```python
from build123d import *

# Parameters (mm, degrees)
F0_R     = 10
F0_W     = 40
F0_H     = 20
F1_DEPTH = 30


with BuildPart() as f1:
    # F0 (on Front) → F1 (new body)
    with BuildSketch(Plane.XZ):
        with BuildLine():
            Line((0, 20), (0, 0))
            Line((0, 0), (110, 0))
            ThreePointArc((110, 0), (117.071068, 2.928932), (120, 10))
            ThreePointArc((120, 10), (122.928932, 17.071068), (130, 20))
            Line((130, 20), (140, 20))
            ThreePointArc((140, 20), (147.071068, 22.928932), (150, 30))
            Line((150, 30), (150, 110))
            ThreePointArc((150, 110), (147.071068, 117.071068), (140, 120))
            Line((140, 120), (130, 120))
            ThreePointArc((130, 120), (122.928932, 122.928932), (120, 130))
            ThreePointArc((120, 130), (117.071068, 137.071068), (110, 140))
            Line((110, 140), (10, 140))
            ThreePointArc((10, 140), (2.928932, 137.071068), (0, 130))
            ThreePointArc((0, 130), (-2.928932, 122.928932), (-10, 120))
            Line((-10, 120), (-40, 120))
            ThreePointArc((-40, 120), (-47.071068, 117.071068), (-50, 110))
            Line((-50, 110), (-50, 30))
            ThreePointArc((-50, 30), (-47.071068, 22.928932), (-40, 20))
            Line((-40, 20), (0, 20))
        make_face()
        with BuildLine():
            Line((-40, 30), (-40, 50))
            Line((-40, 50), (0, 50))
            Line((0, 50), (0, 40))
            ThreePointArc((0, 40), (-2.928932, 32.928932), (-10, 30))
            Line((-10, 30), (-40, 30))
        make_face(mode=Mode.SUBTRACT)
        with BuildLine():
            Line((20, 30), (20, 70))
            Line((20, 70), (100, 70))
            Line((100, 70), (100, 30))
            ThreePointArc((100, 30), (97.071068, 22.928932), (90, 20))
            Line((90, 20), (30, 20))
            ThreePointArc((30, 20), (22.928932, 22.928932), (20, 30))
        make_face(mode=Mode.SUBTRACT)
        with Locations((130, 40)):
            Circle(F0_R, mode=Mode.SUBTRACT)
        with Locations((-20, 70)):
            Rectangle(F0_W, F0_H, mode=Mode.SUBTRACT)
        with BuildLine():
            Line((-40, 90), (-40, 110))
            Line((-40, 110), (-10, 110))
            ThreePointArc((-10, 110), (-2.928932, 107.071068), (0, 100))
            Line((0, 100), (0, 90))
            Line((0, 90), (-40, 90))
        make_face(mode=Mode.SUBTRACT)
        with Locations((130, 70)):
            Circle(F0_R, mode=Mode.SUBTRACT)
        with Locations((130, 100)):
            Circle(F0_R, mode=Mode.SUBTRACT)
        with BuildLine():
            Line((100, 95), (20, 95))
            Line((20, 95), (20, 110))
            ThreePointArc((20, 110), (22.928932, 117.071068), (30, 120))
            Line((30, 120), (90, 120))
            ThreePointArc((90, 120), (97.071068, 117.071068), (100, 110))
            Line((100, 110), (100, 95))
        make_face(mode=Mode.SUBTRACT)
    extrude(amount=F1_DEPTH)


solid = f1.part
```
The model under review builds one solid part; all positions refer to its coordinate system, in mm. A direction names the side the tool comes from. Round coordinates to 2 decimals unless told otherwise and drop trailing zeros. Loops run counter-clockwise (first coordinate to the right, second up) from the corner with the lowest first, then second, coordinate; pieces in that order, holes last.
1) Wall thickness on line 1 along Z through (x, y) = (-16, -9.25); line 2 along Z through (x, y) = (45, -18.25); line 3 along Z through (x, y) = (25, -2): over which ranges is each line inside the solid? List them lowest first.
Values follow:
line 1: z = 20 to 30, 50 to 60, 80 to 90, 110 to 120
line 2: z = 0 to 20, 70 to 95, 120 to 140
line 3: z = 0 to 21.34, 70 to 95, 118.66 to 140
2) Consider section C-C on z = 45.5. State the section outline as (x, y) points.
Values follow:
outline: (-50, -30) - (-40, -30) - (-40, 0) - (-50, 0) - close; (0, -30) - (20, -30) - (20, 0) - (0, 0) - close; (100, -30) - (121.65, -30) - (121.65, 0) - (100, 0) - close; (138.35, -30) - (150, -30) - (150, 0) - (138.35, 0) - close
3) Consider section D-D on z = 117. State the section outline as (x, y) points.
Values follow:
outline: (-47.14, -30) - (22.86, -30) - (22.86, 0) - (-47.14, 0) - close; (97.14, -30) - (147.14, -30) - (147.14, 0) - (97.14, 0) - close
4) The part is to be moulded in two halves that separate along X. For faces 4 (the face through (49, 0, 71)), 5 (the face through (147.15, -14.79, 116.99)), 6 (the face through (0, -15, 95)), say which applies: pulls with the +X half, pulls with the -X half, needs draft (parallel to the pull), parting line crosses it, or undercut.
Values follow:
face 4: needs draft
face 5: pulls with the +X half
face 6: undercut
5) Tool access review of faces 1 (the face through (0, -15, 10)), 2 (the face through (54, -15, 0)), 3 (the face through (0, -15, 45)): name each direction out of +Z, -Z, +X, -X, +Y, -Y from which nothing blocks a thin tool from reaching the whole face with its end or side.
Values follow:
face 1: -Z, -X, +Y, -Y
face 2: -Z, +X, -X, +Y, -Y
face 3: +Y, -Y
6) Clearance check with flat-ended pins moving along their axes: P1, Ø6, axis at y = -9.5, z = 6.5, coming from the -X side; P2, Ø6, axis at x = 75, z = 19.5, coming from the +Y side; P3, Ø9, axis at x = -12, y = -13, coming from the +Z side; P4, Ø2, axis at x = -5, y = -16.5, coming from the -Z side. State where each tip first meets the part, or that it passes through.
Values follow:
P1: stops at x = 0
P2: stops at y = 0
P3: stops at z = 120.32
P4: stops at z = 20
7) Consider section A-A on x = -32. State the section outline as (y, z) points.
Values follow:
outline: (-30, 20) - (0, 20) - (0, 30) - (-30, 30) - close; (-30, 50) - (0, 50) - (0, 60) - (-30, 60) - close; (-30, 80) - (0, 80) - (0, 90) - (-30, 90) - close; (-30, 110) - (0, 110) - (0, 120) - (-30, 120) - close
8) Consider section B-B on x = 71.5. State the section outline as (y, z) points.
Values follow:
outline: (-30, 0) - (0, 0) - (0, 20) - (-30, 20) - close; (-30, 70) - (0, 70) - (0, 95) - (-30, 95) - close; (-30, 120) - (0, 120) - (0, 140) - (-30, 140) - close
